Here's how the part is built. I have some questions about the finished solid (model axes, mm). Coordinates: 2 decimals unless noted, no trailing zeros. Write each loop counter-clockwise with the first axis right and the second up, starting at its lowest first coordinate (ties: lowest second). Pieces come first, ordered by that corner, then holes. Notation, with made-up numbers: (35, -25) -> (55, -25) arc R19 cw to (55, -18) -> close; hole circle Ø4 at (0.5, -26). An arc over 180 degrees is marked (long way). Use a Markdown table: item, result. Add a question column.
Item 1: If we mould it in two halves opening along X, with no side actions, what happens to faces 1 (the cylindrical face through (3.51, 34.97, 3.02)), 2 (the cylindrical face through (-0.1, 38.1, 0.5)), 3 (the flat face through (-6.35, 27, 3)), 4 (the flat face through (3, 27, 5.08))? For each: pulls with the +X half, pulls with the -X half, needs draft (parallel to the pull), parting line crosses it, or undercut.
Item 2: Imagine slicing it at A-A, the plane x = 0. Write out the boundary of the cut face in (y, z) (1 decimal).
Item 3: If I drill on line 1 along Y through (x, z) = (0, 3.8) (1 decimal); line 2 along Z through (x, y) = (5, 25); line 3 along Y through (x, z) = (3.25, 4.8) (3 decimals), over which ranges is the centre line in solid material (lowest first)? Write a range as from..to.
Item 4: Imagine slicing it at D-D, the plane x = -2. Write out the boundary of the cut face in (y, z) (3 decimals).
Item 5: Imagine slicing it at C-C, the plane y = 23.5. Write out the boundary of the cut face in (x, z).
```python
from build123d import *

# Parameters (mm, degrees)
SKETCH1_W           = 12.7
SKETCH1_H           = 53.975
BOSS_EXTRUDE1_DEPTH = 5.08
CUT_EXTRUDE1_DEPTH  = 1.016
SKETCH3_R           = 4.7625
CUT_EXTRUDE2_DEPTH  = 55.498983669


with BuildPart() as part:
    # Sketch1 → Boss-Extrude1 (new body)
    with BuildSketch(Plane.XY):
        with Locations((0, 26.9875)):
            Rectangle(SKETCH1_W, SKETCH1_H)
    extrude(amount=BOSS_EXTRUDE1_DEPTH)

    # Sketch2 → Cut-Extrude1 (cut)
    with BuildSketch(Plane.XY):
        with BuildLine():
            Line((-6.35, -31.75), (-6.35, 31.75))
            ThreePointArc((-6.35, 31.75), (0, 38.1), (6.35, 31.75))
            Line((6.35, 31.75), (6.35, -31.75))
            ThreePointArc((6.35, -31.75), (0, -38.1), (-6.35, -31.75))
        make_face()
    extrude(amount=CUT_EXTRUDE1_DEPTH, mode=Mode.SUBTRACT)

    # Sketch3 → Cut-Extrude2 (cut, through all)
    with BuildSketch(Plane(origin=(0, 0, 1.016), x_dir=(-1, 0, 0), z_dir=(0, 0, -1))):
        with Locations((0, 31.75)):
            Circle(SKETCH3_R)
    extrude(amount=-CUT_EXTRUDE2_DEPTH, mode=Mode.SUBTRACT)


solid = part.part
```
Ans:
| question | item | result |
|---|---|---|
| 1 | face 1 | undercut |
| 1 | face 2 | undercut |
| 1 | face 3 | pulls with the -X half |
| 1 | face 4 | needs draft |
| 2 | outline | (0, 1) -> (27, 1) -> (27, 5.1) -> (0, 5.1) -> close; (36.5, 1) -> (38.1, 1) -> (38.1, 0) -> (54, 0) -> (54, 5.1) -> (36.5, 5.1) -> close |
| 3 | line 1 | y = 0..27, 36.5..54 |
| 3 | line 2 | z = 1.02..5.08 |
| 3 | line 3 | y = 0..28.269, 35.231..53.975 |
| 4 | outline | (0, 1.016) -> (27.428, 1.016) -> (27.428, 5.08) -> (0, 5.08) -> close; (36.072, 1.016) -> (37.777, 1.016) -> (37.777, 0) -> (53.975, 0) -> (53.975, 5.08) -> (36.072, 5.08) -> close |
| 5 | outline | (-6.35, 1.02) -> (6.35, 1.02) -> (6.35, 5.08) -> (-6.35, 5.08) -> close |
